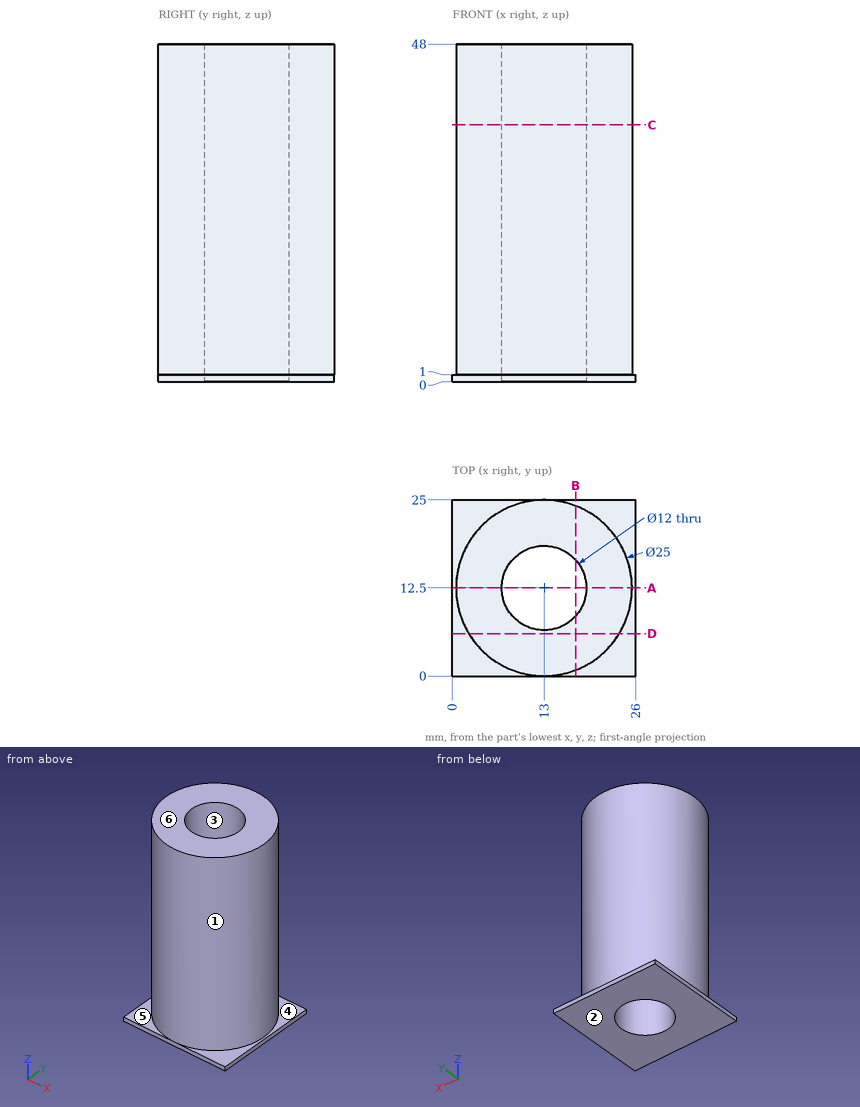
For this review, use the dimensioned drawing (mm, ordinates from the lowest corner) and the shaded views. A direction names the side the tool comes from. Give positions to 0.01 mm unless a question says otherwise; leave off trailing zeros. Order: outer loops, then holes, each group sorted by start corner. A loop starts at its lowest first (then second) coordinate and runs counter-clockwise, first axis right, second up.
1) Take a section at C-C (z = 36.5). Give the boundary of the cut face in (x, y), then the cut area to 3 significant figures.
2) Insertion check: pin 1 (12 mm diameter, centred on x = 3, y = 15.5, fed in from -Z); pin 2 (12 mm diameter, centred on y = 9, z = 42.5, fed in from +X); pin 3 (10 mm diameter, centred on y = 21, z = 20, fed in from -X); pin 4 (1.5 mm diameter, centred on x = 7, z = 30, fed in from +Y). Each pin has a flat end and moves straight along its axis. Give the tip position at first contact, or say it passes through.
3) Take a section at D-D (y = 6). Give the boundary of the cut face in (x, z).
4) For the marked faces 4, 5 and 6, list the 3-axis set-ups (+Z, -Z, +X, -X, +Y, -Y) from which the entire face can be reached by the end or side of a thin tool; tool diameter is ignored.
5) Take a section at B-B (x = 17.5). Give the boundary of the cut face in (y, z).
6) Take a section at A-A (y = 12.5). Give the boundary of the cut face in (x, z), then the cut area to 3 significant figures.
7) The part is to be moulded in two halves that separate along Y. For the marked faces 1, 2 and 3, say which applies: released by +Y, released by -Y, zero draft, split by the parting line, or undercut.
8) Wall thickness on line 1 (Y direction, x = 11.5, z = 15.5); line 2 (X direction, y = 8.25, z = 18.5); line 3 (Y direction, x = 9.5, z = 21.5): over which ranges is each line inside the solid? List them lowest first.
Derived:
1. outline: circle Ø25 at (13, 12.5); hole circle Ø12 at (13, 12.5)
1. area: 378 mm2
2. pin 1: stops at z = 0
2. pin 2: stops at x = 25.5
2. pin 3: stops at x = 1
2. pin 4: stops at y = 23.84
3. outline: (0, 0) - (26, 0) - (26, 1) - (23.68, 1) - (23.68, 48) - (2.32, 48) - (2.32, 1) - (0, 1) - close
4. face 4: +Z, +X
4. face 5: +Z, -X
4. face 6: +Z, +X, -X, +Y, -Y
5. outline: (0, 0) - (8.53, 0) - (8.53, 48) - (0.84, 48) - (0.84, 1) - (0, 1) - close; (16.47, 0) - (25, 0) - (25, 1) - (24.16, 1) - (24.16, 48) - (16.47, 48) - close
6. outline: (0, 0) - (7, 0) - (7, 48) - (0.5, 48) - (0.5, 1) - (0, 1) - close; (19, 0) - (26, 0) - (26, 1) - (25.5, 1) - (25.5, 48) - (19, 48) - close
6. area: 625 mm2
7. face 1: split by the parting line
7. face 2: zero draft
7. face 3: undercut
8. line 1: y = 0.09 to 6.69, 18.31 to 24.91
8. line 2: x = 1.24 to 8.76, 17.24 to 24.76
8. line 3: y = 0.5 to 7.63, 17.37 to 24.5
